Check sheet for the drawn part. Datum: minimum x, y, z corner. Units: mm. A direction names the side the tool comes from. Round coordinates to 2 decimals unless told otherwise and drop trailing zeros. Order: outer loops, then holes, each group sorted by start corner. A loop starts at its lowest first (then second) coordinate and runs counter-clockwise, first axis right, second up.
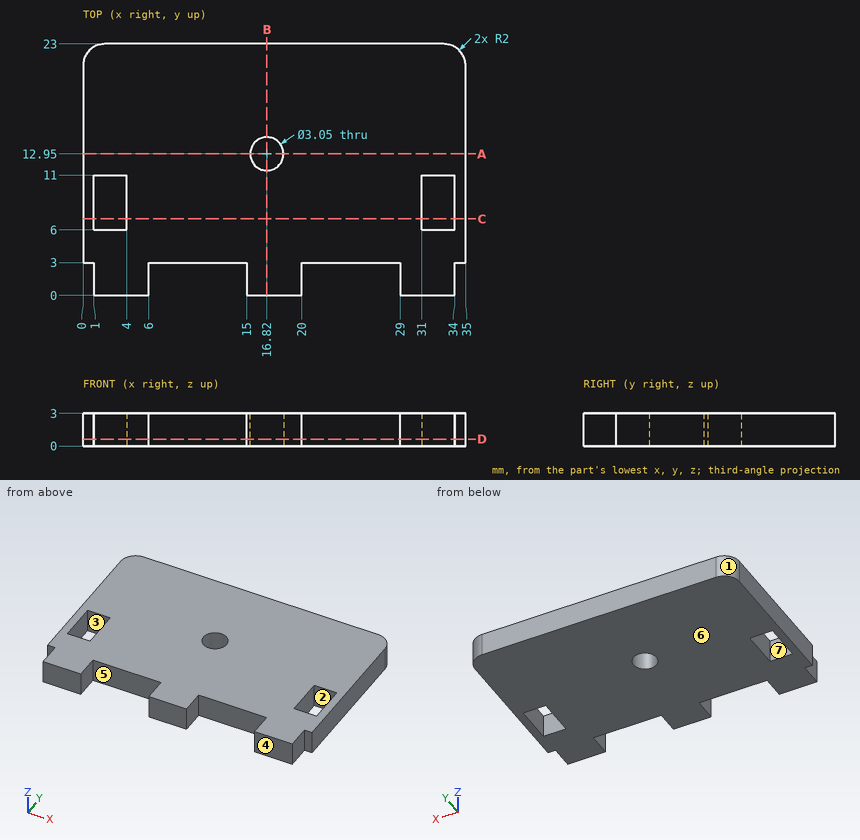
1) Sectioned sample at D-D on z = 0.65. Record the cut outline in (x, y) (3 decimals), and give its area (3 significant figures).
2) Sectioned sample at B-B on x = 16.82. Record the cut outline in (y, z) (3 decimals).
3) Sectioned sample at C-C on y = 7. Record the cut outline in (x, z).
4) Set-up check for the marked faces 5, 6 and 7: record each of +Z, -Z, +X, -X, +Y, -Y from which the full face is reachable in a straight line by a thin tool's end or side.
5) Sectioned sample at A-A on y = 12.95. Record the cut outline in (x, z) (3 decimals).
6) Draft check along X on the marked faces 1, 2, 3 and 4. Enter one of: pulls with the +X half, pulls with the -X half, needs draft (parallel to the pull), parting line crosses it, or undercut.
7) Scan lines: line 1 (X direction, y = 7.5, z = 1.9); line 2 (X direction, y = 2.5, z = 2.35); line 3 (Y direction, x = 16.82, z = 2.05) (3 decimals). Record each from-to range of solid material in increasing order.
8) Gauge pin test, flat ends, axial feed: pin 1 (8 mm diameter, centred on x = 5.5, y = 10.5, fed in from -Z); pin 2 (0.9 mm diameter, centred on x = 11.5, z = 1, fed in from -Y); pin 3 (1.5 mm diameter, centred on y = 1.5, z = 1.5, fed in from -X). Record the tip position at first contact, or that the pin passes through.
Values found:
1. outline: (0, 3) - (1, 3) - (1, 0) - (6, 0) - (6, 3) - (15, 3) - (15, 0) - (20, 0) - (20, 3) - (29, 3) - (29, 0) - (34, 0) - (34, 3) - (35, 3) - (35, 21) arc R2 ccw to (33, 23) - (2, 23) arc R2 ccw to (0, 21) - close; hole (1, 6) - (4, 6) - (4, 11) - (1, 11) - close; hole circle Ø3.05 at (16.82, 12.95); hole (31, 6) - (34, 6) - (34, 11) - (31, 11) - close
1. area: 706 mm2
2. outline: (0, 0) - (11.425, 0) - (11.425, 3) - (0, 3) - close; (14.475, 0) - (23, 0) - (23, 3) - (14.475, 3) - close
3. outline: (0, 0) - (1, 0) - (1, 3) - (0, 3) - close; (4, 0) - (31, 0) - (31, 3) - (4, 3) - close; (34, 0) - (35, 0) - (35, 3) - (34, 3) - close
4. face 5: +Z, -Z, -Y
4. face 6: -Z, +X, -X, +Y, -Y
4. face 7: +Z, -Z
5. outline: (0, 0) - (15.295, 0) - (15.295, 3) - (0, 3) - close; (18.345, 0) - (35, 0) - (35, 3) - (18.345, 3) - close
6. face 1: pulls with the -X half
6. face 2: undercut
6. face 3: undercut
6. face 4: needs draft
7. line 1: x = 0 to 1, 4 to 31, 34 to 35
7. line 2: x = 1 to 6, 15 to 20, 29 to 34
7. line 3: y = 0 to 11.425, 14.475 to 23
8. pin 1: stops at z = 0
8. pin 2: stops at y = 3
8. pin 3: stops at x = 1
